Autodesk Inventor part; units mm, degrees
ref_plane "YZ Plane" through (0, 0, 0) normal (1, 0, 0) x (0, 1, 0)
ref_plane "XZ Plane" through (0, 0, 0) normal (0, 1, 0) x (-1, 0, 0)
ref_plane "XY Plane" through (0, 0, 0) normal (0, 0, 1) x (1, 0, 0)
sketch "構築線" plane through (0, 0, 0) normal (0, 0, 1) x (1, 0, 0)
  circle A0 centre (0, 0) radius 8.5
  circle A1 centre (0, 0) radius 2.8 construction
  circle A2 centre (0, 0) radius 5 construction
  line L0 (0, -8.6) -> (-25, -8.6) construction
  line L1 (0, -11.6) -> (-25, -11.6) construction
  circle A3 centre (-12.8148, 0.95) radius 10.05 construction
  circle A4 centre (-12.8148, 0.95) radius 12.55 construction
  circle A5 centre (0, 5) radius 0.8
  circle A6 centre (-4.3301, 2.5) radius 0.8
  circle A7 centre (-4.3301, -2.5) radius 0.8
  circle A8 centre (0, -5) radius 0.8
  circle A9 centre (4.3301, -2.5) radius 0.8
  circle A10 centre (4.3301, 2.5) radius 0.8
  line L2 (25, -8.6) -> (0, -8.6) construction
  circle A11 centre (12.8148, 0.95) radius 10.05 construction
  circle A12 centre (12.8148, 0.95) radius 12.55 construction
  line L3 (0, -11.6) -> (25, -11.6) construction
  line L4 (-22, -8.6) -> (-22, -2.6)
  arc A13 (-13, 6.4) -> (-22, -2.6) centre (-13, -2.6) ccw
  line L5 (-13, 6.4) -> (-8, 6.4)
  line L6 (-22, -8.6) -> (0, -8.6)
  line L7 (0, 25) -> (0, -25)
  line L8 (0, -8.6) -> (22, -8.6)
  line L9 (22, -8.6) -> (22, -2.6)
  arc A14 (8, 6.4) -> (-8, 6.4) centre (0, 0) ccw
  line L10 (8, 6.4) -> (13, 6.4)
  arc A15 (22, -2.6) -> (13, 6.4) centre (13, -2.6) ccw
  circle A16 centre (0, 0) radius 3
  circle A17 centre (0, 0) radius 1
  circle A18 centre (12.8148, 0.95) radius 1.05
  circle A19 centre (-12.8148, 0.95) radius 1.05
  circle A20 centre (12.8148, 0.95) radius 2.75
  circle A21 centre (-12.8148, 0.95) radius 2.75
  dimension "d0" = 17
  dimension "d1" = 5.6
  dimension "d2" = 10
  dimension "d12" = 25
  dimension "d13" = 8.6
  dimension "d14" = 0
  dimension "d17" = 0
  dimension "d18" = 25
  dimension "d19" = 3
  dimension "d22" = 20.1
  dimension "d23" = 25.1
  dimension "d29" = 1.6
  dimension "d30" = 0
  dimension "d31" = 5
  dimension "d34" = 360
  dimension "d38" = 25
  dimension "d41" = 20.1
  dimension "d42" = 25.1
  dimension "d43" = 25
  dimension "d46" = 22
  dimension "d47" = 6
  dimension "d48" = 5
  dimension "d49" = 50
  dimension "d50" = 25
  dimension "d51" = 25
  dimension "d52" = 22
  dimension "d53" = 6
  dimension "d56" = 15
  dimension "d57" = 15
  dimension "d58" = 6
  dimension "d59" = 2
  dimension "d99" = 2.1
  dimension "d100" = 2.1
  dimension "d105" = 5.5
  dimension "d106" = 5.5
extrude "外形作成" add sketch "構築線" along normal blind 2.5 and the other way blind 1 contours A0 L7 A8 A16 A5 | A0 L7 A14 L10 A15 L9 L8 | L7 A5 A16 A8 A0 | A0 L7 L6 L4 A13 L5 A14 | A16 L7 A17 | L7 A17 A16 | A18 | A19 | A20 | A21
extrude "押し出し4" cut sketch "構築線" against normal blind 1 contours A0 L7 A8 A16 A5 | L7 A5 A16 A8 A0 | A16 L7 A17 | L7 A17 A16
sketch "固定具" plane through (-22, -8.6, 2.5) normal (0, -1, 0) x (1, 0, 0)
  circle A0 centre (6, -1.5) radius 1.05
  line L0 (0, 0) -> (0, -3.5)
  line L1 (0, 0) -> (44, 0)
  circle A1 centre (38, -1.5) radius 1.05
  line L2 (9.15, -0.5) -> (11.15, -0.5)
  line L3 (11.15, -0.5) -> (11.15, -2.5)
  line L4 (11.15, -2.5) -> (9.15, -2.5)
  line L5 (9.15, -2.5) -> (9.15, -0.5)
  line L6 (44, -3.5) -> (0, -3.5)
  line L7 (32.85, -0.5) -> (34.85, -0.5)
  line L8 (34.85, -0.5) -> (34.85, -2.5)
  line L9 (34.85, -2.5) -> (32.85, -2.5)
  line L10 (32.85, -2.5) -> (32.85, -0.5)
  point P0 (22, -2.5)
  dimension "d66" = 2.1
  dimension "d67" = 6
  dimension "d68" = 1.5
  dimension "d69" = 2.1
  dimension "d70" = 32
  dimension "d71" = 1.5
  dimension "d115" = 2
  dimension "d116" = 2
  dimension "d117" = 2.1
  dimension "d118" = 1
  dimension "d119" = 2
  dimension "d120" = 2
  dimension "d121" = 2.1
  dimension "d122" = 1
hole "穴1" at (16, -8.6, 1) direction (0, 1, 0) diameter 1.6 depth 3.5 tip angle 118
hole "穴2" at (-16, -8.6, 1) direction (0, 1, 0) diameter 1.6 depth 3.5 tip angle 118
extrude "押し出し5" cut sketch "構築線" along normal blind 2.1 contours A16 L7 A17 | L7 A17 A16
sketch "スケッチ6" plane through (0, 0, 2.5) normal (0, 0, 1) x (1, 0, 0)
  circle A0 centre (0, 0) radius 1
  circle A1 centre (4.3301, 2.5) radius 0.8
  circle A2 centre (4.3301, -2.5) radius 0.8
  circle A3 centre (0, -5) radius 0.8
  circle A4 centre (-4.3301, -2.5) radius 0.8
  circle A5 centre (-4.3301, 2.5) radius 0.8
  circle A6 centre (0, 5) radius 0.8
  line L0 (-22, -8.6) -> (22, -8.6) construction
  line L1 (22, -8.6) -> (22, -2.6) construction
  arc A7 (22, -2.6) -> (13, 6.4) centre (13, -2.6) ccw construction
  line L2 (13, 6.4) -> (8, 6.4) construction
  arc A8 (8, 6.4) -> (-8, 6.4) centre (0, 0) ccw construction
  line L3 (-8, 6.4) -> (-13, 6.4) construction
  arc A9 (-13, 6.4) -> (-22, -2.6) centre (-13, -2.6) ccw construction
  line L4 (-22, -2.6) -> (-22, -8.6) construction
  line L5 (-22, -7.6) -> (22, -7.6)
  line L6 (-22, -2.6) -> (-22, -8.6)
  line L7 (-22, -7.6) -> (-22, -8.6)
  line L8 (22, -8.6) -> (-22, -8.6)
  line L9 (22, -8.6) -> (22, -7.6)
  dimension "d95" = 44
  dimension "d96" = 1
extrude "押し出し6" add sketch "スケッチ6" along normal blind 0.5 contours L5 L9 L8 L6
extrude "押し出し7" cut sketch "構築線" against normal blind 1 and the other way blind 3 contours A18 | A19
extrude "押し出し8" cut sketch "構築線" along normal blind 1 and the other way blind 1 contours A20
extrude "押し出し9" cut sketch "構築線" along normal blind 1 and the other way blind 1 contours A21
extrude "押し出し10" add sketch "固定具" along normal blind 1 contours L2 L3 L4 L5 | L7 L8 L9 L10
equation "\"d18\" = d12"
properties part number "mount2"
CAD build for the part. Positions are in the model's coordinates, mm. A direction names the side the tool comes from. Round coordinates to 2 decimals unless told otherwise and drop trailing zeros. Order: outer loops, then holes, each group sorted by start corner. A loop starts at its lowest first (then second) coordinate and runs counter-clockwise, first axis right, second up.
Q1. Drop flat-ended pins along their axis: pin 1 (2.5 mm diameter, centred on x = 0, y = 5, fed in from +Z); pin 2 (2 mm diameter, centred on y = 2, z = 1.5, fed in from -X); pin 3 (1 mm diameter, centred on x = 16, z = 1, fed in from -Y); pin 4 (6.5 mm diameter, centred on x = 12.81, y = 0.95, fed in from -Z). Give the stop position or say it passes through.
Q2. Slice it at A-A (x = 0). Write the cut outline in (y, z) (3 decimals).
Q3. Two-plate mould, pull along X, no slides. Class faces 1 (the flat face through (0, -8, 3)), 2 (the flat face through (-1, 1, 2.1)), 3 (the cylindrical face through (-0.129, 10.244, 0.726)): pulls with the +X half, pulls with the -X half, needs draft (parallel to the pull), parting line crosses it, or undercut.
Q4. Which spindle directions (+Z, -Z, +X, -X, +Y, -Y) get a long thin tool onto all of the face, cutting with end or side? Do faces 4 (the flat face through (10, 6.4, 1)), 5 (the flat face through (12, -9, 2)), 6 (the flat face through (-11, 6.4, 1)), 7 (the flat face through (-11.6, 1, 1)), 8 (the flat face through (10.85, -9, 1)). Say none if no direction does.
Q5. Wall check: L1, parallel to Y at x = 0, z = 0.9 (3 decimals); L2, parallel to X at y = -7.5, z = 0.9; L3, parallel to X at y = 2.75, z = 2.4. Give the ranges that are in metal, low to high.
Q6. Slice it at C-C (y = -8). Write the cut outline in (x, z), and give its area (3 significant figures).
Q7. Slice it at D-D (y = 5). Write the cut outline in (x, z), and give its area (3 significant figures).
Q8. Slice it at B-B (y = 2.5). Write the cut outline in (x, z), and give its area (3 significant figures).
Results below:
1. pin 1: stops at z = 2.5
1. pin 2: stops at x = -21.25
1. pin 3: stops at y = -4.92
1. pin 4: stops at z = -1
2. outline: (-8.6, -1) - (-8.5, -1) - (-8.5, 0) - (-5.8, 0) - (-5.8, 2.5) - (-7.6, 2.5) - (-7.6, 3) - (-8.6, 3) - close; (-4.2, 0) - (-3, 0) - (-3, 2.1) - (-1, 2.1) - (-1, 2.5) - (-4.2, 2.5) - close; (1, 2.1) - (3, 2.1) - (3, 0) - (4.2, 0) - (4.2, 2.5) - (1, 2.5) - close; (5.8, 0) - (8.5, 0) - (8.5, -1) - (10.245, -1) - (10.245, 2.5) - (5.8, 2.5) - close
3. face 1: needs draft
3. face 2: undercut
3. face 3: parting line crosses it
4. face 4: +Z, -Z, +X, +Y
4. face 5: +Z, +X, -X, -Y
4. face 6: +Z, -Z, -X, +Y
4. face 7: -Z
4. face 8: +Z, -Z, -Y
5. L1: y = -8.6 to -5.8, -4.2 to -3, 3 to 4.2, 5.8 to 10.245
5. L2: x = -22 to -16.79, -15.21 to 15.21, 16.79 to 22
5. L3: x = -20.24 to -5.09, -3.57 to 3.57, 5.09 to 20.24
6. outline: (-22, -1) - (-2.87, -1) - (-2.87, 0) - (2.87, 0) - (2.87, -1) - (22, -1) - (22, 3) - (-22, 3) - close; hole circle Ø1.6 at (-16, 1); hole circle Ø1.6 at (16, 1)
6. area: 166 mm2
7. outline: (-17.82, -1) - (-6.87, -1) - (-6.87, 0) - (-0.8, 0) - (-0.8, 2.5) - (-17.82, 2.5) - close; (0.8, 0) - (6.87, 0) - (6.87, -1) - (17.82, -1) - (17.82, 2.5) - (0.8, 2.5) - close
7. area: 107 mm2
8. outline: (-20.42, -1) - (-15.09, -1) - (-15.09, 1) - (-10.54, 1) - (-10.54, -1) - (-8.12, -1) - (-8.12, 0) - (-5.13, 0) - (-5.13, 2.5) - (-20.42, 2.5) - close; (-3.53, 0) - (-1.66, 0) - (-1.66, 2.1) - (1.66, 2.1) - (1.66, 0) - (3.53, 0) - (3.53, 2.5) - (-3.53, 2.5) - close; (5.13, 0) - (8.12, 0) - (8.12, -1) - (10.54, -1) - (10.54, 1) - (15.09, 1) - (15.09, -1) - (20.42, -1) - (20.42, 2.5) - (5.13, 2.5) - close
8. area: 93.5 mm2
